Design review of the part built by this model. Coordinates are the model's own, in mm. A direction names the side the tool comes from. Round coordinates to 2 decimals unless told otherwise and drop trailing zeros. Loops run counter-clockwise (first coordinate to the right, second up) from the corner with the lowest first, then second, coordinate; pieces in that order, holes last. Notation, with made-up numbers: (-2.75, 70.25) - (11.25, 70.25) arc R26 ccw to (11.25, 89.25) - close; hole circle Ø6 at (10, 41). An arc over 180 degrees is marked (long way). Return JSON: item names as keys, results as strings. Group by question number.
(1) Clearance check with flat-ended pins moving along their axes: pin 1 (5 mm diameter, centred on y = -29, z = 20, fed in from -X); pin 2 (2 mm diameter, centred on x = 96.5, y = -18, fed in from -Z); pin 3 (3 mm diameter, centred on y = -17, z = 44.5, fed in from -X); pin 4 (1.5 mm diameter, centred on y = -4.5, z = 18.5, fed in from +X). State where each tip first meets the part, or that it passes through.
(2) For faces 5 (the flat face through (2, -20, 0)), 6 (the flat face through (-11, -23, 33)), 7 (the cylindrical face through (-10.648, -8.381, 11.113)), list the 3-axis set-ups (+Z, -Z, +X, -X, +Y, -Y) from which the entire face can be reached by the end or side of a thin tool; tool diameter is ignored.
(3) We need section A-A, the plane z = 25. Write out the cut boundary in (x, y).
(4) The part is to be moulded in two halves that separate along X. For faces 1 (the cylindrical face through (-10.648, -31.381, 11.113)), 2 (the flat face through (-143.49, -20.28, 24.65)), 3 (the flat face through (-2, 0, 47)), 4 (the flat face through (-11, -17, 33)), say which applies: pulls with the +X half, pulls with the -X half, needs draft (parallel to the pull), parting line crosses it, or undercut.
(5) We need section C-C, the plane y = -4. Write out the cut boundary in (x, z), and give its area (3 significant figures).
(6) We need section B-B, the plane x = 0. Write out the cut boundary in (y, z), and give its area (3 significant figures).
(7) Wall thickness on L1, parallel to Z at x = 1, y = -3; L2, parallel to X at y = -12, z = 30.5; L3, parallel to X at y = -20, z = 25: over which ranges is each line inside the solid? List them lowest first. Write a range as [from, to].
from build123d import *

# Parameters (mm, degrees)
BOSS_EXTRUDE1_DEPTH      = 50
CUT_EXTRUDE1_REACH       = 176.66
SKETCH2_R                = 17.5
BOSS_EXTRUDE2_DEPTH      = 3
BOSS_EXTRUDE2_DEPTH_BACK = 3
SKETCH3_R                = 17.5
SKETCH3_R_2              = 12.5


with BuildPart() as part:
    # Sketch1 → Boss-Extrude1 (new body)
    with BuildSketch(Plane.XY):
        Polygon((-162.5, 0), (162.5, 0), (125, -40), (-125, -40), align=None)
    extrude(amount=BOSS_EXTRUDE1_DEPTH)

    # Sketch2 → Cut-Extrude1 (cut, up to next)
    with BuildSketch(Plane(origin=(0, 0, 0), x_dir=(1, 0, 0), z_dir=(0, 1, 0)), mode=Mode.PRIVATE) as cut_extrude1_sk1:
        with Locations(Location((0, -25, 0), (0, 0, 270))):
            Circle(SKETCH2_R)
    cut_extrude1_tool1 = extrude(cut_extrude1_sk1.sketch, amount=-CUT_EXTRUDE1_REACH, mode=Mode.PRIVATE) & part.part
    add(cut_extrude1_tool1.solids().sort_by_distance((0, 0, 25))[0], mode=Mode.SUBTRACT)

    # Sketch3 → Boss-Extrude2 (add, two sides: drawn at the far end of the back side and taken through both)
    with BuildSketch(Plane(origin=(0, -20, 0), x_dir=(1, 0, 0), z_dir=(0, 1, 0)).offset(-BOSS_EXTRUDE2_DEPTH_BACK)):
        with Locations(Location((0, -25, 0), (0, 0, 270))):
            Circle(SKETCH3_R)
        with Locations(Location((0, -25, 0), (0, 0, 270))):
            Circle(SKETCH3_R_2, mode=Mode.SUBTRACT)
    extrude(amount=BOSS_EXTRUDE2_DEPTH + BOSS_EXTRUDE2_DEPTH_BACK)


solid = part.part
Solutions:
{
 "1": {"pin 1": "x = -137.66", "pin 2": "z = 0", "pin 3": "x = -147.97", "pin 4": "x = 158.98"},
 "2": {"face 5": "-Z, +X, -X, +Y, -Y", "face 6": "-Y", "face 7": "+Y"},
 "3": {"outline": "(-162.5, 0) - (-125, -40) - (-17.5, -40) - (-17.5, -23) - (-12.5, -23) - (-12.5, -17) - (-17.5, -17) - (-17.5, 0) - close; (12.5, -23) - (17.5, -23) - (17.5, -40) - (125, -40) - (162.5, 0) - (17.5, 0) - (17.5, -17) - (12.5, -17) - close"},
 "4": {"face 1": "undercut", "face 2": "pulls with the -X half", "face 3": "needs draft", "face 4": "undercut"},
 "5": {"outline": "(-158.75, 0) - (158.75, 0) - (158.75, 50) - (-158.75, 50) - close; hole circle Ø35 at (0, 25)", "area": "14,900 mm^2"},
 "6": {"outline": "(-40, 0) - (0, 0) - (0, 7.5) - (-17, 7.5) - (-17, 12.5) - (-23, 12.5) - (-23, 7.5) - (-40, 7.5) - close; (-40, 42.5) - (-23, 42.5) - (-23, 37.5) - (-17, 37.5) - (-17, 42.5) - (0, 42.5) - (0, 50) - (-40, 50) - close", "area": "660 mm^2"},
 "7": {"L1": "[0, 7.53], [42.47, 50]", "L2": "[-151.25, -16.61], [16.61, 151.25]", "L3": "[-143.75, -12.5], [12.5, 143.75]"}
}
